Verification items for the finished model (mm, model axes). A direction names the side the tool comes from. Round coordinates to 2 decimals unless told otherwise and drop trailing zeros. Write each loop counter-clockwise with the first axis right and the second up, starting at its lowest first coordinate (ties: lowest second). Pieces come first, ordered by that corner, then holes. Notation, with made-up numbers: M 69,-13.5 L 115,-13.5 A10 cw 115,4.5 Z; hole C 15.5,33.25 d3. An arc over 180 degrees is marked long. One line per item, written item: value. Start each with the question number.
Item 1: Section check B-B, the plane y = 17. Record the cut outline in (x, z).
Item 2: Gauge pin test, flat ends, axial feed: pin 1 (1.5 mm diameter, centred on x = 0.5, y = -13, fed in from +Z); pin 2 (3 mm diameter, centred on x = -22.86, y = 22.86, fed in from +Z). Record the tip position at first contact, or that the pin passes through.
Item 3: Section check A-A, the plane z = 10.25. Record the cut outline in (x, y).
Item 4: Thickness scan on probe 1 along X at (y, z) = (22.86, 9.25); probe 2 along X at (y, z) = (-2, 2.25). Record the ranges inside material, lowest first. Write a range as from..to.
Item 5: Tool access check on faces 5 (the face through (-23.47, -21.91, 6.28)), 6 (the face through (26.288, -26.308, 6.439)). Record the directions out of +Z, -Z, +X, -X, +Y, -Y that give a thin tool (end or side, any length) a straight path to the whole face; none if there is none.
Item 6: Draft check along X on faces 1 (the face through (22.66, -22.85, 0.71)), 2 (the face through (-26.67, 0, 6)), 3 (the face through (26.67, 0, 6)), 4 (the face through (-21.084, -21.044, 6.421)). Enter one of: +X half, -X half, draft (parallel to the pull), parting line (faces both ways), or undercut.
from build123d import *

# Parameters (mm, degrees)
F0_W     = 53.34
F0_H     = 53.34
F1_DEPTH = 12.7
F3_D     = 2.2606
F3_DEPTH = 11.43
F3_TIP   = 0.6791527577
F5_DEPTH = 11.43
F4_W     = 50.8
F4_H     = 50.8
F6_DEPTH = 1.27
F7_R     = 1.27


with BuildPart() as f1:
    # F0 (on Top) → F1 (new body)
    with BuildSketch(Plane.XY):
        Rectangle(F0_W, F0_H)
    extrude(amount=F1_DEPTH)

    # F3
    with Locations(Plane.XY.offset(12.7)):
        with Locations((-22.86, 22.86), (22.86, 22.86), (22.86, -22.86), (-22.86, -22.86)):
            Hole(F3_D / 2, depth=F3_DEPTH)
            with Locations((0, 0, -(F3_DEPTH + F3_TIP / 2))):  # 118° drill point
                Cone(0, F3_D / 2, F3_TIP, mode=Mode.SUBTRACT)

    # F2 (on face) → F5 (cut)
    with BuildSketch(Plane.XY.offset(12.7)):
        with BuildLine():
            Line((0, 24.13), (-19.05, 24.13))
            ThreePointArc((-19.05, 24.13), (-19.9480256121, 23.7580256121), (-20.32, 22.86))
            ThreePointArc((-20.32, 22.86), (-21.0639487758, 21.0639487758), (-22.86, 20.32))
            ThreePointArc((-22.86, 20.32), (-23.7580256121, 19.9480256121), (-24.13, 19.05))
            Line((-24.13, 19.05), (-24.13, 0))
            Line((-24.13, 0), (-24.13, -19.05))
            ThreePointArc((-24.13, -19.05), (-23.7580256121, -19.9480256121), (-22.86, -20.32))
            ThreePointArc((-22.86, -20.32), (-21.0639487758, -21.0639487758), (-20.32, -22.86))
            ThreePointArc((-20.32, -22.86), (-19.9480256121, -23.7580256121), (-19.05, -24.13))
            Line((-19.05, -24.13), (0, -24.13))
            Line((0, -24.13), (19.05, -24.13))
            ThreePointArc((19.05, -24.13), (19.9480256121, -23.7580256121), (20.32, -22.86))
            ThreePointArc((20.32, -22.86), (21.0639487758, -21.0639487758), (22.86, -20.32))
            ThreePointArc((22.86, -20.32), (23.7580256121, -19.9480256121), (24.13, -19.05))
            Line((24.13, -19.05), (24.13, 0))
            Line((24.13, 0), (24.13, 19.05))
            ThreePointArc((24.13, 19.05), (23.7580256121, 19.9480256121), (22.86, 20.32))
            ThreePointArc((22.86, 20.32), (21.0639487758, 21.0639487758), (20.32, 22.86))
            ThreePointArc((20.32, 22.86), (19.9480256121, 23.7580256121), (19.05, 24.13))
            Line((19.05, 24.13), (0, 24.13))
        make_face()
    extrude(amount=-F5_DEPTH, mode=Mode.SUBTRACT)

    # F4 (on face) → F6 (cut)
    with BuildSketch(Plane.XY.offset(12.7)):
        Rectangle(F4_W, F4_H)
    extrude(amount=-F6_DEPTH, mode=Mode.SUBTRACT)

    # F7
    f7_edges = [f1.edges().sort_by_distance(p)[0] for p in [
        (-26.67, -26.67, 6.35),
        (26.67, -26.67, 6.35),
        (26.67, 26.67, 6.35),
        (-26.67, 26.67, 6.35),
    ]]
    fillet(f7_edges, radius=F7_R)


solid = f1.part
Response values:
1. outline: M -26.67,0 L 26.67,0 L 26.67,12.7 L 25.4,12.7 L 25.4,11.43 L 24.13,11.43 L 24.13,1.27 L -24.13,1.27 L -24.13,11.43 L -25.4,11.43 L -25.4,12.7 L -26.67,12.7 Z
2. pin 1: stops at z = 1.27
2. pin 2: stops at z = 11.43
3. outline: M -26.67,-25.4 A1.27 ccw -25.4,-26.67 L 25.4,-26.67 A1.27 ccw 26.67,-25.4 L 26.67,25.4 A1.27 ccw 25.4,26.67 L -25.4,26.67 A1.27 ccw -26.67,25.4 Z; hole M -24.13,-19.05 A1.27 ccw -22.86,-20.32 A2.54 cw -20.32,-22.86 A1.27 ccw -19.05,-24.13 L 19.05,-24.13 A1.27 ccw 20.32,-22.86 A2.54 cw 22.86,-20.32 A1.27 ccw 24.13,-19.05 L 24.13,19.05 A1.27 ccw 22.86,20.32 A2.54 cw 20.32,22.86 A1.27 ccw 19.05,24.13 L -19.05,24.13 A1.27 ccw -20.32,22.86 A2.54 cw -22.86,20.32 A1.27 ccw -24.13,19.05 Z; hole C -22.86,-22.86 d2.26; hole C -22.86,22.86 d2.26; hole C 22.86,-22.86 d2.26; hole C 22.86,22.86 d2.26
4. probe 1: x = -26.67..-23.99, -21.73..-20.32, 20.32..21.73, 23.99..26.67
4. probe 2: x = -26.67..-24.13, 24.13..26.67
5. face 5: +Z
5. face 6: +Z, -Z, +X, -Y
6. face 1: undercut
6. face 2: -X half
6. face 3: +X half
6. face 4: undercut
